from build123d import *


with BuildPart() as f1:
    # F0 (on Front) → F1 (revolve)
    with BuildSketch(Plane.XZ):
        with BuildLine():
            Line((0, 66), (0, 0))
            Line((0, 0), (7.05, 0))
            ThreePointArc((7.05, 0), (7.55, 0.2), (8.05, 0))
            Line((8.05, 0), (9.05, 0))
            Line((9.05, 0), (9.05, 61.15))
            ThreePointArc((9.05, 61.15), (8.65, 62.15), (9.05, 63.15))
            Line((9.05, 63.15), (9.05, 65.15))
            Line((9.05, 65.15), (3.5, 65.15))
            Line((3.5, 65.15), (3.5, 65.646447))
            Line((3.5, 65.646447), (3.146447, 66))
            Line((3.146447, 66), (0, 66))
        make_face()
    revolve(axis=Axis((0, 0, 33), (0, 0, 1)))


solid = f1.part
Work out the finished part from the listing and answer in its coordinate system (mm). A direction names the side the tool comes from. Coordinates: 2 decimals unless noted, no trailing zeros. Write each loop counter-clockwise with the first axis right and the second up, starting at its lowest first coordinate (ties: lowest second). Pieces come first, ordered by that corner, then holes. Notation, with made-up numbers: M 8,-17.5 L 61,-17.5 A36 ccw 61,21.5 Z; hole C -14,-33.5 d7. An arc over 180 degrees is marked long. Answer as CSV lines item,"result". Start each with the question number.
Item 1: Flat-ended cylindrical pins translate along their axes: P1, Ø8, axis at y = -5.5, z = 58.5, coming from the +X side; P2, Ø10, axis at y = -6, z = 30, coming from the -X side; P3, Ø5, axis at y = 5, z = 30.5, coming from the -X side. Find the tip coordinate at first contact, or state that the pin passes through.
Item 2: Consider L1, parallel to Z at x = 1, y = 6; L2, parallel to X at y = 0.5, z = 35; L3, parallel to Z at x = 0.5, y = 7.5. Determine where each line is inside the solid, lowest interval first.
Item 3: Section A-A on z = 41.5 is taken. Write down the section's boundary in (x, y).
Item 4: A tool of negligible diameter and unlimited length cuts with its end or side. For faces 1 (the face through (8.63, 2.72, 31)), 2 (the face through (3.233, -1.341, 65.402)), from which of +Z, -Z, +X, -X, +Y, -Y can it reach the whole face along a straight path? Write none if from no direction.
Checks:
1,P1,"stops at x = 8.92"
1,P2,"stops at x = -8.99"
1,P3,"stops at x = -8.7"
2,L1,"z = 0 to 65.15"
2,L2,"x = -9.04 to 9.04"
2,L3,"z = 0.2 to 65.15"
3,outline,"C 0,0 d18.1"
4,face 1,"+Z, -Z"
4,face 2,"+Z"
